```python
from build123d import *

# Parameters (mm, degrees)
CROQUIS1_W                = 59.5
CROQUIS1_H                = 87
CROQUIS1_W_2              = 57.5
CROQUIS1_H_2              = 85
SALIENTE_EXTRUIR1_DEPTH   = 50
SALIENTE_EXTRUIR2_DEPTH   = 10
CROQUIS1_5_R              = 3.25
CROQUIS1_5_R_2            = 2.1
SALIENTE_EXTRUIR3_DEPTH   = 20
SALIENTE_EXTRUIR3_2_DEPTH = 20
CROQUIS2_W                = 59.5
CROQUIS2_H                = 87
SALIENTE_EXTRUIR6_DEPTH   = 2
CROQUIS9_R                = 2.1
CORTAR_EXTRUIR3_DEPTH     = 10
CORTAR_EXTRUIR4_DEPTH     = 100


with BuildPart() as part:
    # Croquis1 → Saliente-Extruir1 (new body)
    with BuildSketch(Plane(origin=(0, 0, 0), x_dir=(1, 0, 0), z_dir=(0, 1, 0))):
        Rectangle(CROQUIS1_W, CROQUIS1_H)
        Rectangle(CROQUIS1_W_2, CROQUIS1_H_2, mode=Mode.SUBTRACT)
    extrude(amount=SALIENTE_EXTRUIR1_DEPTH)

    # Croquis1_4 → Saliente-Extruir2 (add)
    with BuildSketch(Plane(origin=(0, 0, 0), x_dir=(1, 0, 0), z_dir=(0, 1, 0))):
        Polygon((-28.75, -34.5), (-28.75, -35.5), (-14.75, -35.5), (-14.75, 12.5), (-28.75, 12.5), (-28.75, 11.5), (-15.75, 11.5), (-15.75, -34.5), align=None)
    extrude(amount=SALIENTE_EXTRUIR2_DEPTH)



with BuildPart() as body_2:
    # Croquis1_5 → Saliente-Extruir3 (new body)
    with BuildSketch(Plane(origin=(0, 0, 0), x_dir=(1, 0, 0), z_dir=(0, 1, 0))):
        with Locations((19.75, -20)):
            Circle(CROQUIS1_5_R)
        with Locations((19.75, -20)):
            Circle(CROQUIS1_5_R_2, mode=Mode.SUBTRACT)
    extrude(amount=SALIENTE_EXTRUIR3_DEPTH)


with BuildPart() as body_3:
    # Croquis1_5 → Saliente-Extruir3 2 (new body)
    with BuildSketch(Plane(origin=(0, 0, 0), x_dir=(1, 0, 0), z_dir=(0, 1, 0))):
        with Locations((-18.75, 33)):
            Circle(CROQUIS1_5_R)
        with Locations((-18.75, 33)):
            Circle(CROQUIS1_5_R_2, mode=Mode.SUBTRACT)
    extrude(amount=SALIENTE_EXTRUIR3_2_DEPTH)


with BuildPart() as part_1:
    add(part.part)

    add(body_2.part)  # Saliente-Extruir6 merges body 2

    add(body_3.part)  # Saliente-Extruir6 merges body 3
    # Croquis2 → Saliente-Extruir6 (add)
    with BuildSketch(Plane.XZ):
        Rectangle(CROQUIS2_W, CROQUIS2_H)
    extrude(amount=SALIENTE_EXTRUIR6_DEPTH)

    # Croquis9 → Cortar-Extruir3 (cut)
    with BuildSketch(Plane(origin=(0, 0, 0), x_dir=(1, 0, 0), z_dir=(0, 1, 0))):
        with Locations((-18.75, 33)):
            Circle(CROQUIS9_R)
        with Locations((19.75, -20)):
            Circle(CROQUIS9_R)
    extrude(amount=-CORTAR_EXTRUIR3_DEPTH, mode=Mode.SUBTRACT)

    # Croquis10 → Cortar-Extruir4 (cut)
    with BuildSketch(Plane.ZY.offset(29.75)):
        Polygon((0, 39), (14, 39), (14, 36), (-14, 36), (-14, 39), align=None)
    extrude(amount=-CORTAR_EXTRUIR4_DEPTH, mode=Mode.SUBTRACT)


solid = part_1.part
```
Build history of the part. All positions in model axes, mm. A direction names the side the tool comes from. Coordinates: 2 decimals unless noted, no trailing zeros. Write each loop counter-clockwise with the first axis right and the second up, starting at its lowest first coordinate (ties: lowest second). Pieces come first, ordered by that corner, then holes.
1. Drop flat-ended pins along their axis: pin 1 (2 mm diameter, centred on x = 11, z = 6, fed in from +Y); pin 2 (2 mm diameter, centred on x = -18, z = -34.5, fed in from +Y). Give the stop position or say it passes through.
Answer block:
pin 1: stops at y = 0
pin 2: stops at y = 20
2. Drill centre lines: probe 1 along X at (y, z) = (11.5, 20); probe 2 along X at (y, z) = (2.5, 7); probe 3 along X at (y, z) = (13.75, -33). Where is each one in solid material? Low to high.
Answer block:
probe 1: x = -29.75 to -28.75, 16.5 to 17.65, 21.85 to 23, 28.75 to 29.75
probe 2: x = -29.75 to -28.75, -15.75 to -14.75, 28.75 to 29.75
probe 3: x = -29.75 to -28.75, -22 to -20.85, -16.65 to -15.5, 28.75 to 29.75
3. Band-saw the part on B-B, the plane z = -33. Give the cut face in (x, y).
Answer block:
outline: (-29.75, -2) - (-20.85, -2) - (-20.85, 20) - (-22, 20) - (-22, 0) - (-28.75, 0) - (-28.75, 50) - (-29.75, 50) - close; (-16.65, -2) - (29.75, -2) - (29.75, 50) - (28.75, 50) - (28.75, 0) - (-15.5, 0) - (-15.5, 20) - (-16.65, 20) - close
4. 3-axis set-ups, long thin cutter, end or side, ignore diameter. For faces 1 (the flat face through (29.75, 24, -1)), 2 (the flat face through (0, 25, 42.5)): which of +Z, -Z, +X, -X, +Y, -Y reach the whole face in a straight line?
Answer block:
face 1: +Z, -Z, +X, +Y, -Y
face 2: +Y
5. Band-saw the part on A-A, the plane y = 4.5. Give the cut face in (x, z).
Answer block:
outline: (-29.75, -43.5) - (29.75, -43.5) - (29.75, 43.5) - (-29.75, 43.5) - close; circle Ø6.5 at (-18.75, -33); circle Ø6.5 at (19.75, 20); hole (-28.75, -42.5) - (28.75, -42.5) - (28.75, 42.5) - (-28.75, 42.5) - (-28.75, 35.5) - (-14.75, 35.5) - (-14.75, -12.5) - (-28.75, -12.5) - close; hole (-28.75, -11.5) - (-15.75, -11.5) - (-15.75, 34.5) - (-28.75, 34.5) - close; hole circle Ø4.2 at (-18.75, -33); hole circle Ø4.2 at (19.75, 20)
6. Pull direction Z, two halves, no side cores. Call faces 3 (the flat face through (-22, 5, -12.5)), 4 (the flat face through (0, -2, 1)), 5 (the flat face through (0, 24, 43.5)): released by +Z, released by -Z, zero draft, split by the parting line, or undercut.
Answer block:
face 3: undercut
face 4: zero draft
face 5: released by +Z
7. Band-saw the part on C-C, the plane y = 13.5. Give the cut face in (x, z).
Answer block:
outline: (-29.75, -43.5) - (29.75, -43.5) - (29.75, 43.5) - (-29.75, 43.5) - close; circle Ø6.5 at (-18.75, -33); circle Ø6.5 at (19.75, 20); hole (-28.75, -42.5) - (28.75, -42.5) - (28.75, 42.5) - (-28.75, 42.5) - close; hole circle Ø4.2 at (-18.75, -33); hole circle Ø4.2 at (19.75, 20)
8. Band-saw the part on D-D, the plane x = 19.75. Give the cut face in (y, z).
Answer block:
outline: (-2, -43.5) - (50, -43.5) - (50, -42.5) - (0, -42.5) - (0, 16.75) - (20, 16.75) - (20, 17.9) - (-2, 17.9) - close; (-2, 22.1) - (20, 22.1) - (20, 23.25) - (0, 23.25) - (0, 42.5) - (50, 42.5) - (50, 43.5) - (-2, 43.5) - close
